from build123d import *

# Parameters (mm, degrees)
CROQUIS1_W              = 300
CROQUIS1_H              = 180
SALIENTE_EXTRUIR1_DEPTH = 15
CROQUIS2_R              = 2
CORTAR_EXTRUIR1_DEPTH   = 10
CROQUIS3_R              = 3
CROQUIS3_W              = 130
CROQUIS3_H              = 50
CORTAR_EXTRUIR2_DEPTH   = 15
CROQUIS4_R              = 2
CORTAR_EXTRUIR3_DEPTH   = 10


with BuildPart() as part:
    # Croquis1 → Saliente-Extruir1 (new body)
    with BuildSketch(Plane(origin=(0, 0, 0), x_dir=(1, 0, 0), z_dir=(0, 1, 0))):
        Rectangle(CROQUIS1_W, CROQUIS1_H)
    extrude(amount=SALIENTE_EXTRUIR1_DEPTH)

    # Croquis2 → Cortar-Extruir1 (cut)
    with BuildSketch(Plane(origin=(0, 15, 0), x_dir=(1, 0, 0), z_dir=(0, 1, 0))):
        with Locations(Location((-120, -45, 0), (0, 0, 270))):
            Circle(CROQUIS2_R)
        with Locations(Location((-120, -65, 0), (0, 0, 270))):
            Circle(CROQUIS2_R)
        with Locations(Location((120, -45, 0), (0, 0, 270))):
            Circle(CROQUIS2_R)
        with Locations(Location((120, -65, 0), (0, 0, 270))):
            Circle(CROQUIS2_R)
        with Locations(Location((-140, -25, 0), (0, 0, 270))):
            Circle(CROQUIS2_R)
        with Locations(Location((-120, -25, 0), (0, 0, 270))):
            Circle(CROQUIS2_R)
        with Locations(Location((120, -25, 0), (0, 0, 270))):
            Circle(CROQUIS2_R)
        with Locations(Location((140, -25, 0), (0, 0, 270))):
            Circle(CROQUIS2_R)
        with Locations(Location((-120, 65, 0), (0, 0, 270))):
            Circle(CROQUIS2_R)
        with Locations(Location((-120, 45, 0), (0, 0, 270))):
            Circle(CROQUIS2_R)
        with Locations(Location((120, 45, 0), (0, 0, 270))):
            Circle(CROQUIS2_R)
        with Locations(Location((120, 65, 0), (0, 0, 270))):
            Circle(CROQUIS2_R)
    extrude(amount=-CORTAR_EXTRUIR1_DEPTH, mode=Mode.SUBTRACT)

    # Croquis3 → Cortar-Extruir2 (cut)
    with BuildSketch(Plane(origin=(0, 15, 0), x_dir=(1, 0, 0), z_dir=(0, 1, 0))):
        with Locations(Location((110, 65, 0), (0, 0, 270))):
            Circle(CROQUIS3_R)
        Rectangle(CROQUIS3_W, CROQUIS3_H)
    extrude(amount=-CORTAR_EXTRUIR2_DEPTH, mode=Mode.SUBTRACT)

    # Croquis4 → Cortar-Extruir3 (cut)
    with BuildSketch(Plane.XZ):
        with Locations(Location((140, -65, 0), (0, 0, 270))):
            Circle(CROQUIS4_R)
    extrude(amount=-CORTAR_EXTRUIR3_DEPTH, mode=Mode.SUBTRACT)


solid = part.part
Verification items for the finished model (mm, model axes). A direction names the side the tool comes from. Give positions to 0.01 mm unless a question says otherwise; leave off trailing zeros. Loops run counter-clockwise (first coordinate to the right, second up) from the corner with the lowest first, then second, coordinate; pieces in that order, holes last.
1) Draft check along X on faces 1 (the flat face through (-150, 7, 1)), 2 (the flat face through (65, 8, 0)), 3 (the flat face through (150, 7, 1)). Enter one of: pulls with the +X half, pulls with the -X half, needs draft (parallel to the pull), parting line crosses it, or undercut.
2) Sectioned sample at A-A, the plane x = 110. Enter the section's corners in (y, z), then the cut area to 3 significant figures.
3) Set-up check for faces 4 (the flat face through (-65, 8, 0)), 5 (the flat face through (-2, 7, 90)): record each of +Z, -Z, +X, -X, +Y, -Y from which the full face is reachable in a straight line by a thin tool's end or side.
4) Sectioned sample at B-B, the plane y = 2.75. Enter the section's corners in (x, z).
5) Sectioned sample at C-C, the plane x = 21. Enter the section's corners in (y, z), then the cut area to 3 significant figures.
6) Thickness scan on line 1 along X through (y, z) = (6, 44); line 2 along Z through (x, y) = (-58.5, 7.5); line 3 along X through (y, z) = (1.5, -23). Record the ranges inside material, lowest first.
7) Depth check by flat-ended pin: pin 1 Ø6.5 at (x, z) = (-120, 65) entering from +Y; pin 2 Ø2 at (x, z) = (120, 65) entering from +Y. Enter the tip coordinate at first touch or a pass-through.
Answers:
1. face 1: pulls with the -X half
1. face 2: undercut
1. face 3: pulls with the +X half
2. outline: (0, -90) - (15, -90) - (15, -68) - (0, -68) - close; (0, -62) - (15, -62) - (15, 90) - (0, 90) - close
2. area: 2,610 mm2
3. face 4: +Y, -Y
3. face 5: +Z, +X, -X, +Y, -Y
4. outline: (-150, -90) - (150, -90) - (150, 90) - (-150, 90) - close; hole (-65, -25) - (65, -25) - (65, 25) - (-65, 25) - close; hole circle Ø6 at (110, -65); hole circle Ø4 at (140, -65)
5. outline: (0, -90) - (15, -90) - (15, -25) - (0, -25) - close; (0, 25) - (15, 25) - (15, 90) - (0, 90) - close
5. area: 1,950 mm2
6. line 1: x = -150 to -121.73, -118.27 to 118.27, 121.73 to 150
6. line 2: z = -90 to -25, 25 to 90
6. line 3: x = -150 to -65, 65 to 150
7. pin 1: stops at y = 15
7. pin 2: stops at y = 5
